```python
from build123d import *

# Parameters (mm, degrees)
EXTRUDE_1_DEPTH          = 8
SKETCH_2_R               = 1.5
CUT_EXTRUDE_1_DEPTH      = 84.600239234
EXTRUDE_START            = 1
SKETCH_7_R               = 2.5
SKETCH_7_R_2             = 1.5
EXTRUDE_5_DEPTH          = 1
CUT_EXTRUDE_2_DEPTH      = 10
CUT_EXTRUDE_2_DEPTH_BACK = 20
SKETCH_8_R               = 1.5
FILLET_1_R               = 3
FILLET_2_R               = 3


with BuildPart() as part:
    # 草图1 → 凸台-拉伸1 (new body)
    with BuildSketch(Plane.XY):
        Polygon((-29.882727096, 45), (-70, 23), (-70, 5), (-70, -5), (-70, -23), (-30.839658999, -45), (-13, -45), (-13, -8), (-7, -8), (-7, -5), (-13.8744125, -5), (-23.7, -5), (-29.7, -5), (-29.7, -8), (-23.7, -8), (-23.7, -33.722222222), (-26.7, -33.722222222), (-55, -18), (-55, -10), (-55, -5), (-60, -5), (-60, 5), (-55, 5), (-55, 10), (-55, 18), (-26.7, 33.722222222), (-23.7, 33.722222222), (-23.7, 8), (-29.7, 8), (-29.7, 5), (-23.7, 5), (-13.8744125, 5), (-7, 5), (-7, 8.100206116), (-13, 8.100206116), (-13, 45), (-13.841189827, 45), align=None)
    extrude(amount=EXTRUDE_1_DEPTH)

    # 草图2 → 切除-拉伸1 (cut, through all)
    with BuildSketch(Plane.XY.offset(8)):
        with Locations((-62, 17)):
            Circle(SKETCH_2_R)
        with Locations((-62, -17)):
            Circle(SKETCH_2_R)
        with Locations((-18.698729811, 37)):
            Circle(SKETCH_2_R)
        with Locations((-18.698729811, -37)):
            Circle(SKETCH_2_R)
    extrude(amount=-CUT_EXTRUDE_1_DEPTH, mode=Mode.SUBTRACT)

    # 草图7 → 凸台-拉伸5 (add)
    # profile 1 of 2: a face of its own
    with BuildSketch(Plane.XY.offset(8).offset(EXTRUDE_START)):
        with Locations((-18.698729811, 37)):
            Circle(SKETCH_7_R)
        with Locations((-18.698729811, 37)):
            Circle(SKETCH_7_R_2, mode=Mode.SUBTRACT)
    # profile 2 of 2: a face of its own
    with BuildSketch(Plane.XY.offset(8).offset(EXTRUDE_START)):
        with Locations((-18.698729811, -37)):
            Circle(SKETCH_7_R)
        with Locations((-18.698729811, -37)):
            Circle(SKETCH_7_R_2, mode=Mode.SUBTRACT)
    extrude(amount=-EXTRUDE_5_DEPTH)

    # 草图8 → 切除-拉伸2 (cut, two sides: drawn at the far end of the back side and taken through both)
    with BuildSketch(Plane(origin=(0, 8, 0), x_dir=(1, 0, 0), z_dir=(0, 1, 0)).offset(-CUT_EXTRUDE_2_DEPTH_BACK)):
        with Locations(Location((-26.7, -4, 0), (0, 0, 90))):
            Circle(SKETCH_8_R)
        with Locations(Location((-10, -4, 0), (0, 0, 90))):
            Circle(SKETCH_8_R)
    extrude(amount=CUT_EXTRUDE_2_DEPTH + CUT_EXTRUDE_2_DEPTH_BACK, mode=Mode.SUBTRACT)

    # 圆角1
    # the kernel refuses this fillet: 3 mm, written as the material it adds along each edge
    with BuildSketch(Plane(origin=(-55, -18, 0), x_dir=(0.8741572761215378, -0.4856429311786321, 0), z_dir=(0, 0, 1))) as fillet_1_piece_1:
        with BuildLine():
            CenterArc((FILLET_1_R * 0.588403348999, FILLET_1_R), FILLET_1_R, 209.054604099, 60.945395901)
            Line((-FILLET_1_R * 0.285753927123, FILLET_1_R * 0.514357068821), (0, 0))
            Line((0, 0), (FILLET_1_R * 0.588403348999, 0))
        make_face()
    extrude(amount=8)
    with BuildSketch(Plane(origin=(-55, 18, 0), x_dir=(0.8741572761215377, 0.4856429311786323, 0), z_dir=(0, 0, 1))) as fillet_1_piece_2:
        with BuildLine():
            CenterArc((FILLET_1_R * 0.588403348999, -FILLET_1_R), FILLET_1_R, 90, 60.945395901)
            Line((-FILLET_1_R * 0.285753927123, -FILLET_1_R * 0.514357068821), (0, 0))
            Line((0, 0), (FILLET_1_R * 0.588403348999, 0))
        make_face()
    extrude(amount=8)
    with BuildSketch(Plane(origin=(-26.7, -33.722222222, 0), x_dir=(1, 0, 0), z_dir=(0, 0, 1))) as fillet_1_piece_3:
        with BuildLine():
            CenterArc((FILLET_1_R * 0.259126028197, FILLET_1_R), FILLET_1_R, 240.945395901, 29.054604099)
            Line((-FILLET_1_R * 0.226516902981, FILLET_1_R * 0.125842723878), (0, 0))
            Line((0, 0), (FILLET_1_R * 0.259126028197, 0))
        make_face()
    extrude(amount=8)
    with BuildSketch(Plane(origin=(-23.7, -33.722222222, 0), x_dir=(0, 1, 0), z_dir=(0, 0, 1))) as fillet_1_piece_4:
        with BuildLine():
            CenterArc((FILLET_1_R, FILLET_1_R), FILLET_1_R, 180, 90)
            Line((0, FILLET_1_R), (0, 0))
            Line((0, 0), (FILLET_1_R, 0))
        make_face()
    extrude(amount=8)
    with BuildSketch(Plane(origin=(-26.7, 33.722222222, 0), x_dir=(1, 0, 0), z_dir=(0, 0, 1))) as fillet_1_piece_5:
        with BuildLine():
            CenterArc((FILLET_1_R * 0.259126028197, -FILLET_1_R), FILLET_1_R, 90, 29.054604099)
            Line((-FILLET_1_R * 0.226516902981, -FILLET_1_R * 0.125842723878), (0, 0))
            Line((0, 0), (FILLET_1_R * 0.259126028197, 0))
        make_face()
    extrude(amount=8)
    with BuildSketch(Plane(origin=(-23.7, 33.722222222, 0), x_dir=(0, -1, 0), z_dir=(0, 0, 1))) as fillet_1_piece_6:
        with BuildLine():
            CenterArc((FILLET_1_R, -FILLET_1_R), FILLET_1_R, 90, 90)
            Line((0, -FILLET_1_R), (0, 0))
            Line((0, 0), (FILLET_1_R, 0))
        make_face()
    extrude(amount=8)
    # the kernel refuses this fillet: 3 mm, written as the material it takes off along each edge
    with BuildSketch(Plane(origin=(-13, 45, -7.5), x_dir=(-1, 0, 0), z_dir=(0, 0, 1))) as fillet_1_2_piece_1:
        with BuildLine():
            CenterArc((FILLET_1_R, FILLET_1_R), FILLET_1_R, 180, 90)
            Line((0, FILLET_1_R), (0, 0))
            Line((0, 0), (FILLET_1_R, 0))
        make_face()
    extrude(amount=23, mode=Mode.SUBTRACT)
    with BuildSketch(Plane(origin=(-29.882727096, 45, -1.921488827), x_dir=(-0.8768105180064049, -0.48083605887385356, 0), z_dir=(0, 0, 1))) as fillet_1_2_piece_2:
        with BuildLine():
            CenterArc((FILLET_1_R * 0.256198510324, FILLET_1_R), FILLET_1_R, 241.259979418, 28.740020582)
            Line((-FILLET_1_R * 0.22463754855, FILLET_1_R * 0.123189481994), (0, 0))
            Line((0, 0), (FILLET_1_R * 0.256198510324, 0))
        make_face()
    extrude(amount=11.842977655, mode=Mode.SUBTRACT)
    with BuildSketch(Plane(origin=(-13, -45, -7.5), x_dir=(-1, 0, 0), z_dir=(0, 0, 1))) as fillet_1_2_piece_3:
        with BuildLine():
            CenterArc((FILLET_1_R, -FILLET_1_R), FILLET_1_R, 90, 90)
            Line((0, -FILLET_1_R), (0, 0))
            Line((0, 0), (FILLET_1_R, 0))
        make_face()
    extrude(amount=23, mode=Mode.SUBTRACT)
    with BuildSketch(Plane(origin=(-30.839658999, -45, -1.962479999), x_dir=(-0.8718388464587432, 0.4897928396837667, 0), z_dir=(0, 0, 1))) as fillet_1_2_piece_4:
        with BuildLine():
            CenterArc((FILLET_1_R * 0.261663999874, -FILLET_1_R), FILLET_1_R, 90, 29.326966439)
            Line((-FILLET_1_R * 0.22812883981, -FILLET_1_R * 0.128161153541), (0, 0))
            Line((0, 0), (FILLET_1_R * 0.261663999874, 0))
        make_face()
    extrude(amount=11.924959998, mode=Mode.SUBTRACT)
    with BuildSketch(Plane(origin=(-70, -23, -4.389060797), x_dir=(0, 1, 0), z_dir=(0, 0, 1))) as fillet_1_2_piece_5:
        with BuildLine():
            CenterArc((FILLET_1_R * 0.585208106279, -FILLET_1_R), FILLET_1_R, 90, 60.673033561)
            Line((-FILLET_1_R * 0.28663074018, -FILLET_1_R * 0.510207160316), (0, 0))
            Line((0, 0), (FILLET_1_R * 0.585208106279, 0))
        make_face()
    extrude(amount=16.778121594, mode=Mode.SUBTRACT)
    with BuildSketch(Plane(origin=(-70, 23, -4.440787922), x_dir=(0.8768105180064074, 0.48083605887384884, 0), z_dir=(0, 0, 1))) as fillet_1_2_piece_6:
        with BuildLine():
            CenterArc((FILLET_1_R * 0.592105056297, -FILLET_1_R), FILLET_1_R, 90, 61.259979418)
            Line((-FILLET_1_R * 0.284705461709, -FILLET_1_R * 0.519163941126), (0, 0))
            Line((0, 0), (FILLET_1_R * 0.592105056297, 0))
        make_face()
    extrude(amount=16.881575844, mode=Mode.SUBTRACT)

    # 圆角2
    fillet_2_edges = [part.edges().sort_by_distance(p)[0] for p in [
        (-29.7, 6.5, 8),
        (-7, 6.550103058, 8),
        (-7, -6.5, 8),
        (-29.7, -6.5, 8),
        (-7, 6.550103058, 0),
        (-29.7, 6.5, 0),
        (-29.7, -6.5, 0),
        (-7, -6.5, 0),
    ]]
    fillet(fillet_2_edges, radius=FILLET_2_R)


solid = part.part
```
The listing builds one solid part. Answer for the finished solid, in the listing's coordinates (mm). A direction names the side the tool comes from. Give positions to 0.01 mm unless a question says otherwise; leave off trailing zeros. Order: outer loops, then holes, each group sorted by start corner. A loop starts at its lowest first (then second) coordinate and runs counter-clockwise, first axis right, second up. Notation, with made-up numbers: (-10.75, 88.25) -> (27.25, 88.25) arc R18 ccw to (27.25, 110.25) -> close; hole circle Ø4 at (55.25, 88). An arc over 180 degrees is marked (long way). One line per item, written item: value.
1) Find section B-B, the plane z = 4. Count the separate pieces of the cut face and the enclosed holes in it, plus the area to 3 significant figures.
Reported:
separate pieces: 5
enclosed holes: 4
area: 2,440 mm^2
2) Find section C-C, the plane x = -61.5. Determine the outline of the cut face in (y, z).
Reported:
outline: (-27.78, 0) -> (-18.41, 0) -> (-18.41, 8) -> (-27.78, 8) -> close; (-15.59, 0) -> (15.59, 0) -> (15.59, 8) -> (-15.59, 8) -> close; (18.41, 0) -> (27.66, 0) -> (27.66, 8) -> (18.41, 8) -> close
3) Find section A-A, the plane y = -22.5. Determine the outline of the cut face in (x, z).
Reported:
outline: (-69.72, 0) -> (-46.9, 0) -> (-46.9, 8) -> (-69.72, 8) -> close; (-23.7, 0) -> (-13, 0) -> (-13, 8) -> (-23.7, 8) -> close
4) Determine the mould class of faces 5 (the cylindrical face through (-8.67, -6.52, 3.31)), 6 (the cylindrical face through (-28.8, -6.52, 7.14)), 7 (the cylindrical face through (-16.39, -37.96, 8.51)) for opening direction Z: pulls with the +Z half, pulls with the -Z half, needs draft (parallel to the pull), parting line crosses it, or undercut.
Reported:
face 5: undercut
face 6: pulls with the +Z half
face 7: needs draft
5) Find section D-D, the plane y = 37. Determine the outline of the cut face in (x, z).
Reported:
outline: (-44.47, 0) -> (-20.2, 0) -> (-20.2, 9) -> (-21.2, 9) -> (-21.2, 8) -> (-44.47, 8) -> close; (-17.2, 0) -> (-13, 0) -> (-13, 8) -> (-16.2, 8) -> (-16.2, 9) -> (-17.2, 9) -> close
6) A tool of negligible diameter and unlimited length cuts with its end or side. For faces 1 (the flat face through (-13, -25, 4)), 2 (the cylindrical face through (-24.426, 32.679, 3.944)), 3 (the flat face through (-18, -5, 4)), 4 (the cylindrical face through (-27.965, 6.479, 3.194)), from which of +Z, -Z, +X, -X, +Y, -Y can it reach the whole face along a straight path? Write none if from no direction.
Reported:
face 1: +Z, -Z, +X, -Y
face 2: +Z, -Z
face 3: +Z, -Z, +X
face 4: none
7) Flat-ended cylindrical pins translate along their axes: P1, Ø2.5, axis at y = -1, z = 5.5, coming from the +X side; P2, Ø2.5, axis at x = -56.5, z = 4, coming from the -Y side; P3, Ø1.5, axis at y = 19, z = 4, coming from the +X side; P4, Ø1.8, axis at x = -10, z = 4, coming from the -Y side. Find the tip coordinate at first contact, or state that the pin passes through.
Reported:
P1: stops at x = -60
P2: stops at y = -31.29
P3: stops at x = -13
P4: passes through
8) Find the intervals of material crossed by line 1 (X direction, y = 7.15, z = 4); line 2 (X direction, y = 16, z = 0.75); line 3 (X direction, y = -18, z = 2.25), in increasing order.
Reported:
line 1: x = -70 to -55, -29.7 to -28.2, -25.2 to -11.5, -8.5 to -7
line 2: x = -70 to -63.12, -60.88 to -55, -23.7 to -13
line 3: x = -70 to -63.12, -60.88 to -54.43, -23.7 to -13
